from build123d import *

# Parameters (mm, degrees)
F0_R     = 5
F1_DEPTH = 10


with BuildPart() as f1:
    # F0 (on Top) → F1 (new body)
    with BuildSketch(Plane.XY):
        with BuildLine():
            ThreePointArc((0.237756, -7.841041), (5.630434, -5.462296), (7.844645, 0))
            ThreePointArc((7.844645, 0), (5.547002, 5.547002), (0, 7.844645))
            ThreePointArc((0, 7.844645), (-7.844645, 0), (0, -7.844645))
            Line((0, -7.844645), (0.237756, -7.841041))
        make_face()
        Circle(F0_R, mode=Mode.SUBTRACT)
        with BuildLine():
            ThreePointArc((0, 7.844645), (5.547002, 5.547002), (7.844645, 0))
            ThreePointArc((7.844645, 0), (5.630434, -5.462296), (0.237756, -7.841041))
            Line((0.237756, -7.841041), (23.229579, -7.492543))
            ThreePointArc((23.229579, -7.492543), (15.388337, 0.154019), (23.075368, 7.955591))
            Line((23.075368, 7.955591), (0, 7.844645))
        make_face()
        with BuildLine():
            ThreePointArc((30.837062, 0.231125), (28.561446, 5.706325), (23.075368, 7.955591))
            ThreePointArc((23.075368, 7.955591), (15.388337, 0.154019), (23.229579, -7.492543))
            ThreePointArc((23.229579, -7.492543), (28.615828, -5.189411), (30.837062, 0.231125))
        make_face()
        with Locations((22.88138, 0)):
            Circle(F0_R, mode=Mode.SUBTRACT)
    extrude(amount=F1_DEPTH)


solid = f1.part
Source: CAD feature listing. Evaluate the final solid. Frame: model axes, mm. Coordinates: 2 decimals unless noted, no trailing zeros. Write each loop counter-clockwise with the first axis right and the second up, starting at its lowest first coordinate (ties: lowest second). Pieces come first, ordered by that corner, then holes. Notation, with made-up numbers: M 33.5,57.25 L 91.5,57.25 A27 ccw 91.5,73.25 Z; hole C 42.25,-34 d9. An arc over 180 degrees is marked long. Use a Markdown table: item, result.
1) Ray query, L1, parallel to X at y = 4, z = 3.25; L2, parallel to X at y = -0.25, z = 4.5; L3, parallel to Y at x = 20.5, z = 9.25. Return the intervals inside material, ascending.
Conclusion:
| item | result |
|---|---|
| L1 | x = -6.75 to -3, 3 to 19.88, 25.88 to 29.86 |
| L2 | x = -7.84 to -4.99, 4.99 to 17.89, 27.88 to 30.82 |
| L3 | y = -7.53 to -4.4, 4.4 to 7.94 |
2) Section C-C, the plane y = -3.25. Output: boundary loops of the cut face in (x, z), then the cut area to 3 significant figures.
Conclusion:
| item | result |
|---|---|
| outline | M -7.14,0 L -3.8,0 L -3.8,10 L -7.14,10 Z; M 3.8,0 L 19.08,0 L 19.08,10 L 3.8,10 Z; M 26.68,0 L 30.01,0 L 30.01,10 L 26.68,10 Z |
| area | 219 mm^2 |
3) Mould query, pull axis Y, two halves, no side actions, for faces 1 (the cylindrical face through (-1.08, -4.88, 4.93)), 2 (the flat face through (11, 0, 10)), 3 (the cylindrical face through (-7.843, 0.172, 4.93)). Classes: pulls with the +Y half, pulls with the -Y half, needs draft (parallel to the pull), parting line crosses it, or undercut.
Conclusion:
| item | result |
|---|---|
| face 1 | undercut |
| face 2 | needs draft |
| face 3 | parting line crosses it |
4) Section A-A, the plane z = 2.5. Output: boundary loops of the cut face in (x, y), then the cut area to 3 significant figures.
Conclusion:
| item | result |
|---|---|
| outline | M 0,-7.84 L 0.24,-7.84 L 23.23,-7.49 A7.72 ccw 23.08,7.96 L 0,7.84 A7.84 ccw Z; hole C 0,0 d10; hole C 22.88,0 d10 |
| area | 393 mm^2 |
5) First-contact query: pin 1 Ø2 at (x, z) = (-0.5, 4.5) entering from +Y; pin 2 Ø5 at (x, z) = (22.5, 2) entering from -Y; pin 3 Ø6 at (x, z) = (26.5, 1.5) entering from +Y. Flat tips, straight axial feed; report the tip coordinate or a pass-through.
Conclusion:
| item | result |
|---|---|
| pin 1 | stops at y = 7.85 |
| pin 2 | stops at y = -7.54 |
| pin 3 | stops at y = 7.95 |
6) Section D-D, the plane y = 6.25. Output: boundary loops of the cut face in (x, z).
Conclusion:
| item | result |
|---|---|
| outline | M -4.74,0 L 27.95,0 L 27.95,10 L -4.74,10 Z |
7) Section B-B, the plane x = 21.5. Output: boundary loops of the cut face in (y, z).
Conclusion:
| item | result |
|---|---|
| outline | M -7.52,0 L -4.81,0 L -4.81,10 L -7.52,10 Z; M 4.81,0 L 7.95,0 L 7.95,10 L 4.81,10 Z |
